The listing builds one solid part. Answer for the finished solid, in the listing's coordinates (mm). Give positions to 0.01 mm unless a question says otherwise; leave off trailing zeros. Loops run counter-clockwise (first coordinate to the right, second up) from the corner with the lowest first, then second, coordinate; pieces in that order, holes last.
Item 1: Each of these flat-tipped pins is pushed along its axis until it touches: pin 1 Ø5.5 at (x, z) = (-10, -2) entering from +Y; pin 2 Ø1.5 at (x, y) = (-50, 1) entering from -Z. Where does it stop, or does it pass through?
Item 2: Section B-B, the plane x = -10 is taken. Give the vertices of the cut face in (y, z), and give its area (3 significant figures).
Item 3: Section D-D, the plane x = -61 is taken. Give the vertices of the cut face in (y, z), and give its area (3 significant figures).
Item 4: Section C-C, the plane x = -92.5 is taken. Give the vertices of the cut face in (y, z) (3 decimals), and give its area (3 significant figures).
Item 5: Section A-A, the plane y = 1.6 is taken. Give the vertices of the cut face in (x, z).
Item 6: Consider line 1 along Z through (x, y) = (-85, 1.8); line 2 along Z through (x, y) = (-9.5, 2.95); line 3 along Z through (x, y) = (-74.5, 2.4). Determine where each line is inside the solid, lowest interval first.
Autodesk Inventor part; units mm, degrees
ref_plane "YZ Plane" through (0, 0, 0) normal (1, 0, 0) x (0, 1, 0)
ref_plane "XZ Plane" through (0, 0, 0) normal (0, 1, 0) x (-1, 0, 0)
ref_plane "XY Plane" through (0, 0, 0) normal (0, 0, 1) x (1, 0, 0)
sketch "スケッチ1" plane through (0, 0, 0) normal (0, 1, 0) x (-1, 0, 0)
  arc A0 (120.7701, -0.6068) -> (119.8564, 3.2634) centre (120.103, 1.2786) ccw
  arc A1 (41.4452, -14.9694) -> (120.7701, -0.6068) centre (36.8758, 236.5065) ccw
  arc A2 (30.7183, -14.8468) -> (41.4452, -14.9694) centre (38.1525, 166.2425) ccw
  arc A3 (11.0166, -11.3447) -> (30.7183, -14.8468) centre (33.77, 59.49) ccw
  arc A4 (-0.3565, -5.7585) -> (11.0166, -11.3447) centre (24.3575, 30.1875) ccw
  arc A5 (-3.5852, -2.6234) -> (-0.3565, -5.7585) centre (7.25, 5.305) ccw
  arc A6 (-0.7848, 4.3726) -> (-3.5852, -2.6234) centre (0, 0) ccw
  arc A7 (7.6183, 5.1344) -> (-0.7848, 4.3726) centre (7.775, -43.32) ccw
  arc A8 (35.5607, 3.8888) -> (7.6183, 5.1344) centre (8.565, -287.665) ccw
  arc A9 (35.5607, 3.8888) -> (52.6853, 2.3311) centre (526.9475, 5310.875) ccw
  arc A10 (52.6853, 2.3311) -> (84.6244, 0.9905) centre (82.86, 340.0849) ccw
  arc A11 (84.6244, 0.9905) -> (119.8564, 3.2634) centre (83.0725, 299.245) ccw
extrude "押し出し1" add sketch "スケッチ1" along normal blind 4
sketch "スケッチ2" plane through (0, 0, 0) normal (0, -1, 0) x (1, 0, 0)
  circle A0 centre (-10, -2) radius 3
  circle A1 centre (-85, -5) radius 3
  point P0 (0, 0)
  dimension "d3" = 6
  dimension "d4" = 6
  dimension "d5" = 10
  dimension "d6" = 2
  dimension "d7" = 5
  dimension "d8" = 85
extrude "押し出し2" cut sketch "スケッチ2" against normal through all
thicken "厚み1" operation cut thickness 1 both sides no extend neighbours no toward (-0.2771555, 0, 0.9608251) faces at (-13.1498, 2.6667, -11.9948) (-9.6787, 1.3333, -10.8909) (-35.4848, 2.6667, -14.9797) (-114.3801, 1.3333, -2.7717) (-121.1079, 2.6667, 3.0079) (0.7651, 1.3333, -5.4662) (1.1102, 2.6667, 4.3015) (-0.1407, 1.3333, 4.5295) (-23.1571, 2.6667, 4.7721) (-45.0737, 2.6667, 3.0166) (-70.4143, 2.6667, 1.2143) (-115.9582, 2.6667, 2.8049)
equation "\"d4\" = d3"
properties part number "plate_sf2" material "木材 (オーク)"
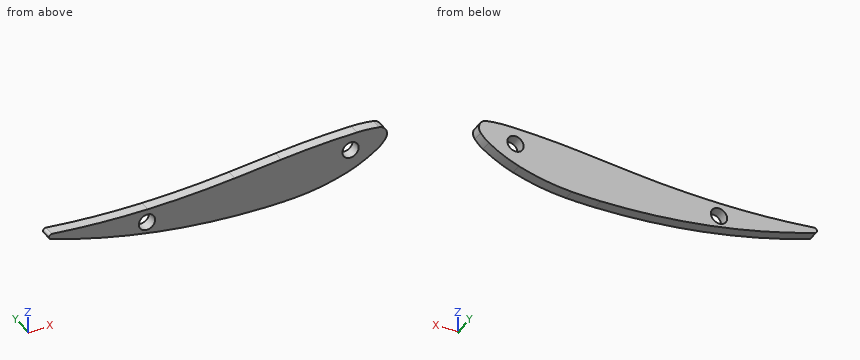
Worked answers:
1. pin 1: passes through
1. pin 2: stops at z = -13.71
2. outline: (0, -9.94) - (4, -9.94) - (4, -5) - (0, -5) - close; (0, 1) - (4, 1) - (4, 4.13) - (0, 4.13) - close
2. area: 32.3 mm2
3. outline: (0, -12.85) - (4, -12.85) - (4, 0.69) - (0, 0.69) - close
3. area: 54.1 mm2
4. outline: (0, -7.758) - (4, -7.758) - (4, 0.135) - (0, 0.135) - close
4. area: 31.6 mm2
5. outline: (-120.44, 0.34) arc R250.51 ccw to (-41.43, -13.97) arc R180.22 ccw to (-30.76, -13.85) arc R73.4 ccw to (-11.32, -10.39) arc R42.63 ccw to (-0.21, -4.93) arc R12.42 ccw to (2.78, -2.03) arc R3.44 ccw to (0.61, 3.39) arc R47.46 ccw to (-7.62, 4.13) arc R291.8 ccw to (-35.47, 2.89) arc R5311.23 cw to (-52.6, 1.34) arc R340.09 cw to (-84.63, -0.01) arc R299.26 cw to (-119.98, 2.27) arc R1 ccw to start; hole circle Ø6 at (-85, -5); hole circle Ø6 at (-10, -2)
6. line 1: z = -9.35 to -8, -2 to -0.01
6. line 2: z = -9.76 to -4.96, 0.96 to 4.13
6. line 3: z = -11.17 to 0.09
